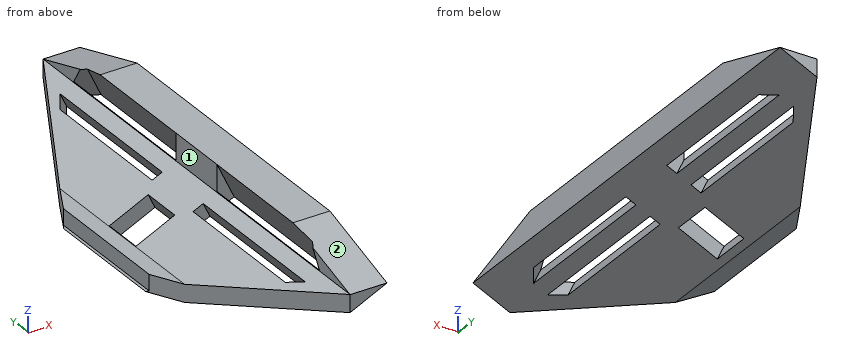
Solid Edge part; units mm, degrees
sketch "Sketch1" plane through (0, 0, 0) normal (1, 0, 0) x (0, 1, 0)
  line L0 (-150, -25) -> (150, -25)
  line L1 (150, -25) -> (150, 25)
  line L2 (150, 25) -> (-150, 25)
  line L3 (-150, 25) -> (-150, -25)
  dimension "D1" = 150
  dimension "D2" = 150
extrude "Protrusion1" add sketch "Sketch1" along normal mid plane 80
sketch "Sketch2" plane through (40, 0, 0) normal (1, 0, 0) x (0, 1, 0)
  line L0 (-150, 7.9) -> (-94.21, 25)
  line L1 (-94.21, 25) -> (94.21, 25)
  line L2 (94.21, 25) -> (150, 7.9)
  dimension "D1" = 94.21
  dimension "D2" = 150
extrude "Cutout1" cut sketch "Sketch2" against normal through all material side at (40, -122.1197, 16.4978)
sketch "Sketch3" plane through (0, -150, -8.55) normal (0, -1, 0) x (1, 0, 0)
  line L0 (-30, -16.45) -> (40, 16.41)
  dimension "D1" = 30
  dimension "D2" = 40
extrude "Cutout2" cut sketch "Sketch3" against normal through all material side at (5.0212, -150, -8.6153)
sketch "Sketch4" plane through (0, -150, -8.55) normal (0, -1, 0) x (1, 0, 0)
  line L0 (16.7577, 33.55) -> (16.7577, 16.55)
  line L1 (16.7577, 16.55) -> (-30, -5.4027)
  line L2 (-30, -5.4027) -> (-40, -5.4027)
  dimension "D1" = 16.7577
  dimension "D2" = 30
extrude "Cutout3" cut sketch "Sketch4" against normal through all material side at (16.7077, -150, 16.5)
sketch "Sketch5" plane through (0, -150, -8.55) normal (0, -1, 0) x (1, 0, 0)
  line L0 (-40, -16.45) -> (-41, -16.45)
  line L1 (-41, -16.45) -> (-40, -15.45)
  dimension "D1" = 40
extrude "Extrusionsausprägung_2" add sketch "Sketch5" against normal blind 300 material side at (-40.5, -150, -24.95)
sketch "Sketch6" plane through (28.3789, 0, 25) normal (0, 0, 1) x (0, -1, 0)
  line L0 (-150, -11.6211) -> (-40, -69.3789)
  line L1 (-40, -69.3789) -> (40, -69.3789)
  line L2 (150, -11.6211) -> (40, -69.3789)
  line L3 (150, 11.6211) -> (150, -11.6211)
  line L4 (-150, 11.6211) -> (150, 11.6211)
  line L5 (-150, 11.6211) -> (-150, -11.6211)
  dimension "D1" = 40
  dimension "D2" = 150
extrude "Cutout4" cut sketch "Sketch6" against normal through all flip side to cut
sketch "Sketch7" plane through (5, 0, -8.57) normal (0.4249, 0, -0.9052) x (0, 1, 0)
  line L0 (-109.9992, 24.9085) -> (-119.9992, 17.9088)
  line L1 (-119.9992, 17.9088) -> (-19.9992, 17.9088)
  line L2 (-19.9992, 17.9088) -> (-19.9992, 24.9085)
  line L3 (-19.9992, 24.9085) -> (-109.9992, 24.9085)
  line L4 (-19.9992, 8.0688) -> (-119.9992, 8.0688)
  line L5 (-109.9992, 1.0688) -> (-119.9992, 8.0688)
  line L6 (-19.9992, 1.0688) -> (-109.9992, 1.0688)
  line L7 (-19.9992, 8.0688) -> (-19.9992, 1.0688)
  dimension "D1" = 19.9992
  dimension "D2" = 119.9992
  dimension "D3" = 19.9992
extrude "Cutout5" cut sketch "Sketch7" against normal through all
mirror "Mirror1" about plane through (0, 0, 0) normal (0, -1, 0) of "Cutout5"
sketch "Sketch8" plane through (5, 0, -8.57) normal (0.4249, 0, -0.9052) x (0, 1, 0)
  line L0 (-13, -33.6667) -> (13, -33.6667)
  line L1 (13, -33.6667) -> (13, -6.6667)
  line L2 (13, -6.6667) -> (-13, -6.6667)
  line L3 (-13, -6.6667) -> (-13, -33.6667)
  dimension "D1" = 13
  dimension "D2" = 13
extrude "Cutout7" cut sketch "Sketch8" against normal through all
extrude "Protrusion2" [suppressed]
Check sheet for the modelled part. Datum: model origin and axes. Units: mm. Face numbers are marked on the shaded views. A direction names the side the tool comes from. Give positions to 0.01 mm unless a question says otherwise; leave off trailing zeros. Write each loop counter-clockwise with the first axis right and the second up, starting at its lowest first coordinate (ties: lowest second). Pieces come first, ordered by that corner, then holes.
Item 1: Cross-section at D-D (y = -105.5). Enter the section's corners in (x, z), and give its area (3 significant figures).
Item 2: Scan lines: L1, parallel to X at y = 125.5, z = 13; L2, parallel to X at y = 86, z = -3; L3, parallel to Z at x = 24.5, y = -55.5. Record each from-to range of solid material in increasing order.
Item 3: Gauge pin test, flat ends, axial feed: pin 1 (10.5 mm diameter, centred on x = -15.5, z = -14.5, fed in from +Y); pin 2 (11 mm diameter, centred on x = -37, y = -10.5, fed in from +Z); pin 3 (1 mm diameter, centred on x = 6, y = 21, fed in from -Z); pin 4 (5 mm diameter, centred on x = -26, z = -7.5, fed in from -Y). Record the tip position at first contact, or that the pin passes through.
Item 4: Cross-section at C-C (y = 101.5). Enter the section's corners in (x, z) (1 decimal), and give its area (3 significant figures).
Item 5: Cross-section at B-B (x = -14.5). Enter the section's corners in (y, z).
Item 6: Cross-section at A-A (y = -28). Enter the section's corners in (x, z), and give its area (3 significant figures).
Item 7: Access from +Z, -Z, +X, -X, +Y, -Y to the whole of each face (thin tool, end or side, straight path). Record for the marked faces 1 and 2.
Report:
1. outline: (-6.61, -14.02) - (5.97, -8.12) - (1.72, 0.94) - (-6.61, -2.97) - close; (8.05, 3.91) - (12.3, -5.14) - (21.21, -0.96) - (16.76, 8.53) - (16.76, 8) - close; (18.38, 21.54) - (27.55, 2.01) - (40, 7.86) - (40, 21.54) - close
1. area: 510 mm2
2. L1: x = 16.76 to 40
2. L2: x = -6.67 to 3.57, 11.3 to 16.87
2. L3: z = 8.51 to 25
3. pin 1: stops at y = 98.56
3. pin 2: stops at z = -13.95
3. pin 3: stops at z = -8.34
3. pin 4: passes through
4. outline: (-8.7, -15) - (6, -8.1) - (1.7, 0.9) - (-8.7, -4) - close; (8.1, 3.9) - (12.3, -5.1) - (21.2, -1) - (16.8, 8.5) - (16.8, 8) - close; (17.8, 22.8) - (27.5, 2) - (40, 7.9) - (40, 22.8) - close
4. area: 560 mm2
5. outline: (-90.47, -17.72) - (-13, -17.72) - (-13, -6.68) - (-90.47, -6.68) - close; (13, -17.72) - (90.47, -17.72) - (90.47, -6.68) - (13, -6.68) - close
6. outline: (-41, -25) - (-30, -25) - (5.97, -8.12) - (1.72, 0.94) - (-30, -13.95) - (-40, -13.95) - (-40, -24) - close; (8.05, 3.91) - (12.3, -5.14) - (21.21, -0.96) - (16.76, 8.53) - (16.76, 8) - close; (16.76, 25) - (27.55, 2.01) - (40, 7.86) - (40, 25) - close
6. area: 957 mm2
7. face 1: +Z, -X, +Y, -Y
7. face 2: +Z, +X, -X, -Y
